```python
from build123d import *

# Parameters (mm, degrees)
SKETCH1_R           = 3.5
BOSS_EXTRUDE1_DEPTH = 5
SKETCH2_R           = 4
BOSS_EXTRUDE2_DEPTH = 5
SKETCH3_R           = 3.5
BOSS_EXTRUDE3_DEPTH = 100


with BuildPart() as part:
    # Sketch1 → Boss-Extrude1 (new body)
    with BuildSketch(Plane(origin=(0, 0, 0), x_dir=(1, 0, 0), z_dir=(0, 1, 0))):
        with Locations(Location((0, 0, 0), (0, 0, 270))):  # turned: the seam where the file's is
            Circle(SKETCH1_R)
    extrude(amount=BOSS_EXTRUDE1_DEPTH)

    # Sketch2 → Boss-Extrude2 (add)
    with BuildSketch(Plane(origin=(0, 5, 0), x_dir=(1, 0, 0), z_dir=(0, 1, 0))):
        with Locations(Location((0, 0, 0), (0, 0, 270))):  # turned: the seam where the file's is
            Circle(SKETCH2_R)
    extrude(amount=BOSS_EXTRUDE2_DEPTH)

    # Sketch3 → Boss-Extrude3 (add)
    with BuildSketch(Plane(origin=(0, 10, 0), x_dir=(1, 0, 0), z_dir=(0, 1, 0))):
        with Locations(Location((0, 0, 0), (0, 0, 270))):  # turned: the seam where the file's is
            Circle(SKETCH3_R)
    extrude(amount=BOSS_EXTRUDE3_DEPTH)


solid = part.part
```
Model file for the job. Use its own axes, mm. A direction names the side the tool comes from. Coordinates: 2 decimals unless noted, no trailing zeros. Order: outer loops, then holes, each group sorted by start corner. A loop starts at its lowest first (then second) coordinate and runs counter-clockwise, first axis right, second up. Notation, with made-up numbers: (2, 72.5) - (61, 72.5) arc R8 cw to (61, 84.5) - close; hole circle Ø5 at (1.5, 25). An arc over 180 degrees is marked (long way). Return JSON: item names as keys, results as strings. Group by question number.
1) Saw through at C-C, the plane y = 65. Write the cut outline in (x, z), plus the area to 3 significant figures.
2) Saw through at B-B, the plane x = 0. Write the cut outline in (y, z), plus the area to 3 significant figures.
3) Saw through at A-A, the plane z = 0. Write the cut outline in (x, y).
4) Probe line 1 (X direction, y = 75, z = 0.25); line 2 (Y direction, x = -3.5, z = 1); line 3 (X direction, y = 87, z = 1.5). List the from-to ranges inside material, lowest first. Write a range as from..to.
5) Flat gauge pins, fed straight in: P1, Ø2, axis at x = -2.5, y = 18, coming from the +Z side; P2, Ø2, axis at x = -1, y = 18.5, coming from the +Z side. Where does each tip first touch, or does it go through?
6) Tool access for faces 1 (the cylindrical face through (-3.417, 2.465, -0.759)), 2 (the cylindrical face through (-3.417, 59.3, -0.759)), 3 (the flat face through (0, 0, 0)): list every direction of +Z, -Z, +X, -X, +Y, -Y with a clear straight run to the whole face (end or side of a thin tool).
Values found:
{
 "1": {"outline": "circle Ø7 at (0, 0)", "area": "38.5 mm²"},
 "2": {"outline": "(0, -3.5) - (5, -3.5) - (5, -4) - (10, -4) - (10, -3.5) - (110, -3.5) - (110, 3.5) - (10, 3.5) - (10, 4) - (5, 4) - (5, 3.5) - (0, 3.5) - close", "area": "775 mm²"},
 "3": {"outline": "(-4, 5) - (-3.5, 5) - (-3.5, 0) - (3.5, 0) - (3.5, 5) - (4, 5) - (4, 10) - (3.5, 10) - (3.5, 110) - (-3.5, 110) - (-3.5, 10) - (-4, 10) - close"},
 "4": {"line 1": "x = -3.49..3.49", "line 2": "y = 5..10", "line 3": "x = -3.16..3.16"},
 "5": {"P1": "stops at z = 3.16", "P2": "stops at z = 3.5"},
 "6": {"face 1": "-Y", "face 2": "+Y", "face 3": "+Z, -Z, +X, -X, -Y"}
}
